Autodesk Inventor part; units mm, degrees
ref_plane "YZ Plane" through (0, 0, 0) normal (1, 0, 0) x (0, 1, 0)
ref_plane "XZ Plane" through (0, 0, 0) normal (0, 1, 0) x (-1, 0, 0)
ref_plane "XY Plane" through (0, 0, 0) normal (0, 0, 1) x (1, 0, 0)
sketch "Sketch3" plane through (0, 0, 0) normal (0, 1, 0) x (-1, 0, 0)
  arc A0 (127.5964, -8.854) -> (151.8036, -8.854) centre (139.7, -12.7) ccw
  arc A1 (0, -12.7) -> (279.4, -12.7) centre (139.7, -12.7) ccw
  line L0 (279.4, -12.7) -> (279.4, 0)
  line L1 (279.4, 0) -> (151.8036, 0)
  line L2 (151.8036, 0) -> (151.8036, -8.854)
  line L3 (127.5964, 0) -> (0, 0)
  line L4 (0, 0) -> (0, -12.7)
  line L5 (127.5964, 0) -> (127.5964, -8.854)
  point P0 (0, -12.7)
  dimension "d9" = 279.4
extrude "Extrusion2" add sketch "Sketch3" along normal blind 2.54
sketch "Sketch4" plane through (0, 2.54, 0) normal (0, 1, 0) x (1, 0, 0)
  arc A0 (-127.5964, 8.854) -> (-151.8036, 8.854) centre (-139.7, 12.7) ccw
  arc A1 (0, 12.7) -> (-279.4, 12.7) centre (-139.7, 12.7) ccw
  line L0 (-127.5964, 0) -> (0, 0)
  line L1 (0, 0) -> (2.54, 0)
  line L2 (-279.4, 12.7) -> (-279.4, 0)
  line L3 (-279.4, 0) -> (-281.94, 0)
  circle A2 centre (-139.7, 12.7) radius 142.8058
  line L4 (0, 0) -> (2.54, 0)
  line L5 (0, 0) -> (0, 12.7)
  arc A3 (0, 12.7) -> (-279.4, 12.7) centre (-139.7, 12.7) ccw
  line L6 (-279.4, 0) -> (-279.4, 12.7)
  line L7 (-279.4, 0) -> (-281.94, 0)
  dimension "d12" = 2.54
  dimension "d13" = 2.54
extrude "Extrusion3" add sketch "Sketch4" along normal blind 25.4 contours A1 L2 L3 A2 L1 L5 picked at (-280.1039, 19.3593)
sketch "Sketch6" plane through (-279.4, 0, -12.7) normal (-1, 0, 0) x (0, 0, 1)
  line L0 (12.7, 0) -> (3.846, 0)
  line L1 (0, 2.54) -> (-139.7, 2.54)
  line L2 (12.7, 0) -> (-25.4, 0)
  line L3 (-25.4, 0) -> (-25.4, 2.54)
  line L4 (-25.4, 2.54) -> (12.7, 2.54)
  line L5 (12.7, 2.54) -> (12.7, 0)
  dimension "d16" = 38.1
extrude "Extrusion4" add sketch "Sketch6" along normal mid plane 76.2
sketch "Sketch7" plane through (0, 0, 0) normal (1, 0, 0) x (0, 0, -1)
  line L0 (38.1, 0) -> (0, 0)
  line L1 (0, 0) -> (38.1, 0)
  line L2 (38.1, 0) -> (38.1, 2.54)
  line L3 (38.1, 2.54) -> (0, 2.54)
  line L4 (0, 2.54) -> (0, 0)
  dimension "d19" = 38.1
  dimension "d20" = 2.54
extrude "Extrusion5" add sketch "Sketch7" along normal mid plane 76.2
properties part number "FlatRotationalTransfer"
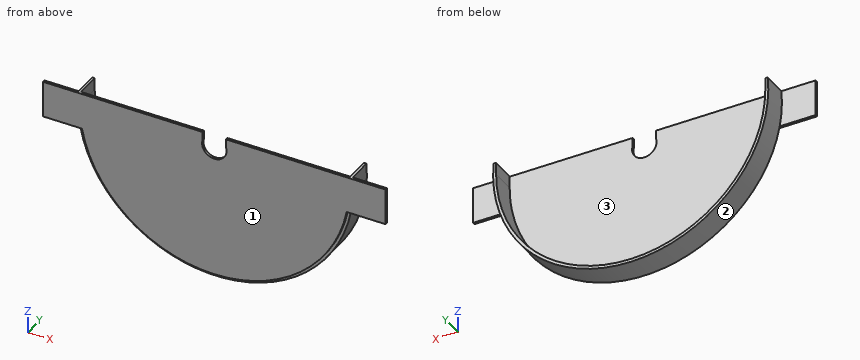
Read the model definition and answer for the solid it produces. Units are mm, in the model's axes. Face numbers are marked on the shaded views. Round coordinates to 2 decimals unless told otherwise and drop trailing zeros.
1) Straight lines are drawn through the part: L1, parallel to X at y = 20.25, z = -13; L2, parallel to X at y = 0.85, z = -12.7; L3, parallel to Y at x = -185, z = -46. For each, find the intervals that lie inside material, in ascending order.
2) Flat-ended cylindrical pins translate along their axes: pin 1 (5 mm diameter, centred on x = -238, y = 10.5, fed in from -Z); pin 2 (10 mm diameter, centred on y = 16, z = -7.5, fed in from +X); pin 3 (4 mm diameter, centred on x = -241, z = -100.5, fed in from +Y); pin 4 (12 mm diameter, centred on x = -44.5, z = -101.5, fed in from -Y). Find the tip coordinate at first contact, or state that the pin passes through.
3) The mould has two halves that part along X. Classify the marked faces 1, 2 and 3: released by +X, released by -X, zero draft, split by the parting line, or undercut.
Resolved:
1. L1: x = -282.51 to -279.4, 0 to 3.11
1. L2: x = -317.5 to -152.4, -127 to 38.1
1. L3: y = 0 to 2.54
2. pin 1: stops at z = -118.6
2. pin 2: stops at x = 3.11
2. pin 3: stops at y = 2.54
2. pin 4: stops at y = 0
3. face 1: zero draft
3. face 2: split by the parting line
3. face 3: undercut
